```python
from build123d import *

# Parameters (mm, degrees)
SKETCH1_W           = 135
SKETCH1_H           = 150
BOSS_EXTRUDE1_DEPTH = 5
CUT_EXTRUDE1_REACH  = 103.026
SKETCH2_R           = 4
CUT_EXTRUDE5_REACH  = 103.026
SKETCH6_R           = 4
CUT_EXTRUDE6_REACH  = 103.026
SKETCH7_R           = 2


with BuildPart() as part:
    # Sketch1 → Boss-Extrude1 (new body)
    with BuildSketch(Plane.XY):
        Rectangle(SKETCH1_W, SKETCH1_H)
    extrude(amount=BOSS_EXTRUDE1_DEPTH)

    # Sketch2 → Cut-Extrude1 (cut, up to next)
    with BuildSketch(Plane.XY.offset(5), mode=Mode.PRIVATE) as cut_extrude1_sk1:
        with Locations((-57.5, 65)):
            Circle(SKETCH2_R)
    cut_extrude1_tool1 = extrude(cut_extrude1_sk1.sketch, amount=-CUT_EXTRUDE1_REACH, mode=Mode.PRIVATE) & part.part
    # Sketch2 → Cut-Extrude1 (cut, up to next)
    with BuildSketch(Plane.XY.offset(5), mode=Mode.PRIVATE) as cut_extrude1_sk2:
        with Locations((-57.5, -25)):
            Circle(SKETCH2_R)
    cut_extrude1_tool2 = extrude(cut_extrude1_sk2.sketch, amount=-CUT_EXTRUDE1_REACH, mode=Mode.PRIVATE) & part.part
    # Sketch2 → Cut-Extrude1 (cut, up to next)
    with BuildSketch(Plane.XY.offset(5), mode=Mode.PRIVATE) as cut_extrude1_sk3:
        with BuildLine():
            Line((37.5, 69), (47.5, 69))
            ThreePointArc((47.5, 69), (51.5, 65), (47.5, 61))
            Line((47.5, 61), (37.5, 61))
            ThreePointArc((37.5, 61), (33.5, 65), (37.5, 69))
        make_face()
    cut_extrude1_tool3 = extrude(cut_extrude1_sk3.sketch, amount=-CUT_EXTRUDE1_REACH, mode=Mode.PRIVATE) & part.part
    # Sketch2 → Cut-Extrude1 (cut, up to next)
    with BuildSketch(Plane.XY.offset(5), mode=Mode.PRIVATE) as cut_extrude1_sk4:
        with BuildLine():
            Line((37.5, -29), (47.5, -29))
            ThreePointArc((47.5, -29), (51.5, -25), (47.5, -21))
            Line((47.5, -21), (37.5, -21))
            ThreePointArc((37.5, -21), (33.5, -25), (37.5, -29))
        make_face()
    cut_extrude1_tool4 = extrude(cut_extrude1_sk4.sketch, amount=-CUT_EXTRUDE1_REACH, mode=Mode.PRIVATE) & part.part
    add(cut_extrude1_tool1.solids().sort_by_distance((-57.5, 65, 5))[0], mode=Mode.SUBTRACT)
    add(cut_extrude1_tool2.solids().sort_by_distance((-57.5, -25, 5))[0], mode=Mode.SUBTRACT)
    add(cut_extrude1_tool3.solids().sort_by_distance((42.5, 65, 5))[0], mode=Mode.SUBTRACT)
    add(cut_extrude1_tool4.solids().sort_by_distance((42.5, -25, 5))[0], mode=Mode.SUBTRACT)

    # Sketch6 → Cut-Extrude5 (cut, up to next)
    with BuildSketch(Plane.XY.offset(5), mode=Mode.PRIVATE) as cut_extrude5_sk1:
        with Locations((-60.5, 23)):
            Circle(SKETCH6_R)
    cut_extrude5_tool1 = extrude(cut_extrude5_sk1.sketch, amount=-CUT_EXTRUDE5_REACH, mode=Mode.PRIVATE) & part.part
    # Sketch6 → Cut-Extrude5 (cut, up to next)
    with BuildSketch(Plane.XY.offset(5), mode=Mode.PRIVATE) as cut_extrude5_sk2:
        with Locations((-60.5, -45)):
            Circle(SKETCH6_R)
    cut_extrude5_tool2 = extrude(cut_extrude5_sk2.sketch, amount=-CUT_EXTRUDE5_REACH, mode=Mode.PRIVATE) & part.part
    # Sketch6 → Cut-Extrude5 (cut, up to next)
    with BuildSketch(Plane.XY.offset(5), mode=Mode.PRIVATE) as cut_extrude5_sk3:
        with Locations((41.5, 23)):
            Circle(SKETCH6_R)
    cut_extrude5_tool3 = extrude(cut_extrude5_sk3.sketch, amount=-CUT_EXTRUDE5_REACH, mode=Mode.PRIVATE) & part.part
    # Sketch6 → Cut-Extrude5 (cut, up to next)
    with BuildSketch(Plane.XY.offset(5), mode=Mode.PRIVATE) as cut_extrude5_sk4:
        with Locations((41.5, -45)):
            Circle(SKETCH6_R)
    cut_extrude5_tool4 = extrude(cut_extrude5_sk4.sketch, amount=-CUT_EXTRUDE5_REACH, mode=Mode.PRIVATE) & part.part
    add(cut_extrude5_tool1.solids().sort_by_distance((-60.5, 23, 5))[0], mode=Mode.SUBTRACT)
    add(cut_extrude5_tool2.solids().sort_by_distance((-60.5, -45, 5))[0], mode=Mode.SUBTRACT)
    add(cut_extrude5_tool3.solids().sort_by_distance((41.5, 23, 5))[0], mode=Mode.SUBTRACT)
    add(cut_extrude5_tool4.solids().sort_by_distance((41.5, -45, 5))[0], mode=Mode.SUBTRACT)

    # Sketch7 → Cut-Extrude6 (cut, up to next)
    with BuildSketch(Plane(origin=(0, 0, 0), x_dir=(-1, 0, 0), z_dir=(0, 0, -1)), mode=Mode.PRIVATE) as cut_extrude6_sk1:
        with Locations((-63.5, 47.5)):
            Circle(SKETCH7_R)
    cut_extrude6_tool1 = extrude(cut_extrude6_sk1.sketch, amount=-CUT_EXTRUDE6_REACH, mode=Mode.PRIVATE) & part.part
    # Sketch7 → Cut-Extrude6 (cut, up to next)
    with BuildSketch(Plane(origin=(0, 0, 0), x_dir=(-1, 0, 0), z_dir=(0, 0, -1)), mode=Mode.PRIVATE) as cut_extrude6_sk2:
        with Locations((-53.5, 47.5)):
            Circle(SKETCH7_R)
    cut_extrude6_tool2 = extrude(cut_extrude6_sk2.sketch, amount=-CUT_EXTRUDE6_REACH, mode=Mode.PRIVATE) & part.part
    # Sketch7 → Cut-Extrude6 (cut, up to next)
    with BuildSketch(Plane(origin=(0, 0, 0), x_dir=(-1, 0, 0), z_dir=(0, 0, -1)), mode=Mode.PRIVATE) as cut_extrude6_sk3:
        with Locations((-64, 17)):
            Circle(SKETCH7_R)
    cut_extrude6_tool3 = extrude(cut_extrude6_sk3.sketch, amount=-CUT_EXTRUDE6_REACH, mode=Mode.PRIVATE) & part.part
    # Sketch7 → Cut-Extrude6 (cut, up to next)
    with BuildSketch(Plane(origin=(0, 0, 0), x_dir=(-1, 0, 0), z_dir=(0, 0, -1)), mode=Mode.PRIVATE) as cut_extrude6_sk4:
        with Locations((-53, 17)):
            Circle(SKETCH7_R)
    cut_extrude6_tool4 = extrude(cut_extrude6_sk4.sketch, amount=-CUT_EXTRUDE6_REACH, mode=Mode.PRIVATE) & part.part
    add(cut_extrude6_tool1.solids().sort_by_distance((63.5, 47.5, 0))[0], mode=Mode.SUBTRACT)
    add(cut_extrude6_tool2.solids().sort_by_distance((53.5, 47.5, 0))[0], mode=Mode.SUBTRACT)
    add(cut_extrude6_tool3.solids().sort_by_distance((64, 17, 0))[0], mode=Mode.SUBTRACT)
    add(cut_extrude6_tool4.solids().sort_by_distance((53, 17, 0))[0], mode=Mode.SUBTRACT)


solid = part.part
```
Work out the finished part from the listing and answer in its coordinate system (mm). A direction names the side the tool comes from. Give positions to 0.01 mm unless a question says otherwise; leave off trailing zeros. Loops run counter-clockwise (first coordinate to the right, second up) from the corner with the lowest first, then second, coordinate; pieces in that order, holes last. Notation, with made-up numbers: (6, 73) -> (15, 73) arc R27 ccw to (15, 112) -> close; hole circle Ø2 at (-29, 41). An arc over 180 degrees is marked (long way). Write item = value, one per line. Start each with the question number.
(1) Find section C-C on y = 47.5. Give the vertices of the cut face in (x, z).
(2) Find section B-B on z = 1. Give the number of separate pieces and of enclosed holes in the cut face, and give its area (3 significant figures).
(3) The mould has two halves that part along Y. Classify faces 1 (the flat face through (-1, -75, 2)), 2 (the cylindrical face through (40.979, 26.966, 2.535)), 3 (the flat face through (-1, 75, 2)): +Y half, -Y half, draft (parallel to the pull), parting line (faces both ways), or undercut.
(4) Find section A-A on y = 23. Give the vertices of the cut face in (x, z).
(5) Find the intervals of material crossed by probe 1 along Y at (x, z) = (41.5, 2.25); probe 2 along Y at (x, z) = (63.5, 1.25); probe 3 along X at (y, z) = (20.5, 3.3), in increasing order. Write a range as from..to.
(6) Which of the six approach directions +Z, -Z, +X, -X, +Y, -Y give full straight-line access (tool end or side, diameter ignored) to faces 4 (the flat face through (-1, 1, 0)), 5 (the flat face through (43, 61, 3))?
From the geometry:
q1.outline = (-67.5, 0) -> (51.5, 0) -> (51.5, 5) -> (-67.5, 5) -> close; (55.5, 0) -> (61.5, 0) -> (61.5, 5) -> (55.5, 5) -> close; (65.5, 0) -> (67.5, 0) -> (67.5, 5) -> (65.5, 5) -> close
q2.separate_pieces = 1
q2.enclosed_holes = 12
q2.area = 19,600 mm^2
q3.face_1 = -Y half
q3.face_2 = undercut
q3.face_3 = +Y half
q4.outline = (-67.5, 0) -> (-64.5, 0) -> (-64.5, 5) -> (-67.5, 5) -> close; (-56.5, 0) -> (37.5, 0) -> (37.5, 5) -> (-56.5, 5) -> close; (45.5, 0) -> (67.5, 0) -> (67.5, 5) -> (45.5, 5) -> close
q5.probe_1 = -75..-49, -41..-29, -21..19, 27..61, 69..75
q5.probe_2 = -75..15.06, 18.94..45.5, 49.5..75
q5.probe_3 = -67.5..-63.62, -57.38..38.38, 44.62..67.5
q6.face_4 = -Z, +X, -X, +Y, -Y
q6.face_5 = +Z, -Z
